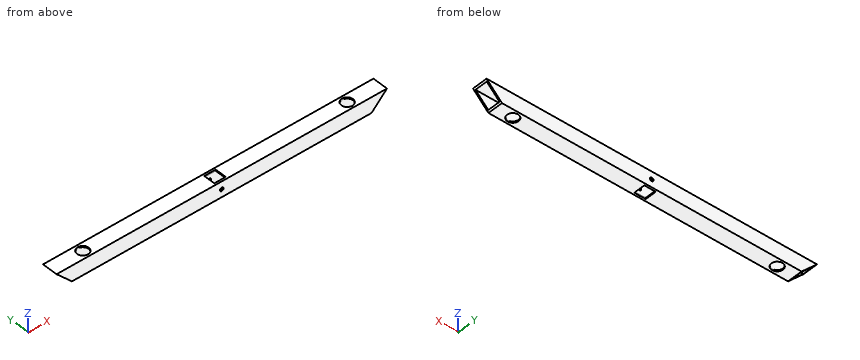
from build123d import *

# Parameters (mm, degrees)
BOSS_EXTRUDE1_DEPTH = 35
SHELL1_T            = -3
SKETCH4_R           = 13
CUT_EXTRUDE1_DEPTH  = 49
SKETCH5_W           = 26
SKETCH5_H           = 26
CUT_EXTRUDE2_DEPTH  = 39
SKETCH6_R           = 4
CUT_EXTRUDE3_DEPTH  = 35


with BuildPart() as part:
    # Sketch1 → Boss-Extrude1 (new body)
    with BuildSketch(Plane(origin=(0, 0, 0), x_dir=(1, 0, 0), z_dir=(0, 1, 0))):
        Polygon((-325, -12.5), (-290, 22.5), (390, 22.5), (425, -12.5), align=None)
    extrude(amount=BOSS_EXTRUDE1_DEPTH)

    # Shell1
    shell1_openings = [part.faces().sort_by_distance(p)[0] for p in [
        (-307.5, 17.5, -5),
        (407.5, 17.5, -5),
    ]]
    offset(amount=SHELL1_T, openings=shell1_openings, kind=Kind.INTERSECTION)

    # Sketch4 → Cut-Extrude1 (cut)
    with BuildSketch(Plane.XY.offset(12.5)):
        with Locations((-250, 17.5)):
            Circle(SKETCH4_R)
        with Locations((350, 17.5)):
            Circle(SKETCH4_R)
    extrude(amount=-CUT_EXTRUDE1_DEPTH, mode=Mode.SUBTRACT)

    # Sketch5 → Cut-Extrude2 (cut)
    with BuildSketch(Plane(origin=(0, 0, -22.5), x_dir=(-1, 0, 0), z_dir=(0, 0, -1))):
        with Locations((-50, 17.5)):
            Rectangle(SKETCH5_W, SKETCH5_H)
    extrude(amount=-CUT_EXTRUDE2_DEPTH, mode=Mode.SUBTRACT)

    # Sketch6 → Cut-Extrude3 (cut)
    with BuildSketch(Plane(origin=(0, 35, 0), x_dir=(1, 0, 0), z_dir=(0, 1, 0))):
        with Locations((50, 5)):
            Circle(SKETCH6_R)
    extrude(amount=-CUT_EXTRUDE3_DEPTH, mode=Mode.SUBTRACT)


solid = part.part
Work out the finished part from the listing and answer in its coordinate system (mm). Coordinates: 2 decimals unless noted, no trailing zeros. Order: outer loops, then holes, each group sorted by start corner. A loop starts at its lowest first (then second) coordinate and runs counter-clockwise, first axis right, second up. Notation, with made-up numbers: (23.25, 69.25) - (65.25, 69.25) arc R11 ccw to (65.25, 80.25) - close; hole circle Ø7 at (-27.75, -34). An arc over 180 degrees is marked (long way). Put each result on its own line as item: value. Start each with the question number.
1) Find section A-A (x = 127.5). Give the vertices of the cut face in (y, z).
2) Find section C-C (x = -250). Give the vertices of the cut face in (y, z), plus the area to 3 significant figures.
3) Find the intervals of material crossed by line 1 (Y direction, x = 192.5, z = -18); line 2 (Z direction, x = -237, y = 15.5); line 3 (Y direction, x = -250, z = -21), in increasing order. Write a range as from..to.
4) Find section D-D (x = 346). Give the vertices of the cut face in (y, z), plus the area to 3 significant figures.
5) Find section B-B (y = 23). State how many separate pieces and enclosed holes the cut face has, plus the area to 3 significant figures.
6) Flat-ended cylindrical pins translate along their axes: pin 1 (2.5 mm diameter, centred on x = 50.5, z = 11, fed in from -Y); pin 2 (0.9 mm diameter, centred on y = 22, z = -20.5, fed in from +X); pin 3 (1.5 mm diameter, centred on y = 19, z = -21.5, fed in from -X); pin 4 (2.5 mm diameter, centred on y = 11.5, z = 11.5, fed in from -X). Find the tip coordinate at first contact, or state that the pin passes through.
Results list:
1. outline: (0, -22.5) - (35, -22.5) - (35, 12.5) - (0, 12.5) - close; hole (3, -19.5) - (32, -19.5) - (32, 9.5) - (3, 9.5) - close
2. outline: (0, -22.5) - (4.5, -22.5) - (4.5, -19.5) - (3, -19.5) - (3, 9.5) - (4.5, 9.5) - (4.5, 12.5) - (0, 12.5) - close; (30.5, -22.5) - (35, -22.5) - (35, 12.5) - (30.5, 12.5) - (30.5, 9.5) - (32, 9.5) - (32, -19.5) - (30.5, -19.5) - close
2. area: 228 mm^2
3. line 1: y = 0..3, 32..35
3. line 2: z = -22.5..-19.5, 9.5..12.5
3. line 3: y = 0..4.5, 30.5..35
4. outline: (0, -22.5) - (5.13, -22.5) - (5.13, -19.5) - (3, -19.5) - (3, 9.5) - (5.13, 9.5) - (5.13, 12.5) - (0, 12.5) - close; (29.87, -22.5) - (35, -22.5) - (35, 12.5) - (29.87, 12.5) - (29.87, 9.5) - (32, 9.5) - (32, -19.5) - (29.87, -19.5) - close
4. area: 236 mm^2
5. separate pieces: 8
5. enclosed holes: 0
5. area: 3,850 mm^2
6. pin 1: stops at y = 0
6. pin 2: stops at x = 392.45
6. pin 3: stops at x = -291.75
6. pin 4: stops at x = -325
